The listing builds one solid part. Answer for the finished solid, in the listing's coordinates (mm). A direction names the side the tool comes from. Coordinates: 2 decimals unless noted, no trailing zeros. Order: outer loops, then holes, each group sorted by start corner. A loop starts at its lowest first (then second) coordinate and runs counter-clockwise, first axis right, second up. Notation, with made-up numbers: (48.5, -7) - (74.5, -7) arc R11 ccw to (74.5, 11) - close; hole circle Ø11 at (81, 10.25). An arc over 180 degrees is marked (long way). One line per item, written item: value. Start each with the question number.
```python
from build123d import *

# Parameters (mm, degrees)
F0_R     = 5
F1_DEPTH = 25
F2_DEPTH = 25


with BuildPart() as f1:
    # F0 (on Top) → F1 (new body)
    with BuildSketch(Plane.XY):
        with BuildLine():
            Line((-37.271081, -27.341548), (27.728919, -27.341548))
            Line((27.728919, -27.341548), (27.728919, -12.341548))
            Line((27.728919, -12.341548), (38.254101, 0))
            Line((38.254101, 0), (29.131456, 6.146329))
            Line((29.131456, 6.146329), (16.831115, -3.876174))
            Line((16.831115, -3.876174), (10.514384, 3.876174))
            Line((10.514384, 3.876174), (22.142908, 13.35127))
            Line((22.142908, 13.35127), (14.383989, 22.100874))
            Line((14.383989, 22.100874), (2.728919, 12.658452))
            Line((2.728919, 12.658452), (-7.271081, 12.658452))
            Line((-7.271081, 12.658452), (-7.271081, 2.658452))
            Line((-7.271081, 2.658452), (-12.271081, 2.658452))
            Line((-12.271081, 2.658452), (-12.271081, 12.658452))
            Line((-12.271081, 12.658452), (-32.271081, 12.658452))
            Line((-32.271081, 12.658452), (-32.271081, -7.341548))
            Line((-32.271081, -7.341548), (-37.271081, -7.341548))
            ThreePointArc((-37.271081, -7.341548), (-40.806615, -8.806014), (-42.271081, -12.341548))
            Line((-42.271081, -12.341548), (-42.271081, -22.341548))
            ThreePointArc((-42.271081, -22.341548), (-40.806615, -25.877082), (-37.271081, -27.341548))
        make_face()
        with Locations((-8.769282, -11.614208)):
            Circle(F0_R, mode=Mode.SUBTRACT)
    extrude(amount=F1_DEPTH)

    # F0 (on Top) → F2 (join)
    with BuildSketch(Plane.XY):
        with BuildLine():
            Line((-37.271081, -27.341548), (27.728919, -27.341548))
            Line((27.728919, -27.341548), (27.728919, -12.341548))
            Line((27.728919, -12.341548), (38.254101, 0))
            Line((38.254101, 0), (29.131456, 6.146329))
            Line((29.131456, 6.146329), (16.831115, -3.876174))
            Line((16.831115, -3.876174), (10.514384, 3.876174))
            Line((10.514384, 3.876174), (22.142908, 13.35127))
            Line((22.142908, 13.35127), (14.383989, 22.100874))
            Line((14.383989, 22.100874), (2.728919, 12.658452))
            Line((2.728919, 12.658452), (-7.271081, 12.658452))
            Line((-7.271081, 12.658452), (-7.271081, 2.658452))
            Line((-7.271081, 2.658452), (-12.271081, 2.658452))
            Line((-12.271081, 2.658452), (-12.271081, 12.658452))
            Line((-12.271081, 12.658452), (-32.271081, 12.658452))
            Line((-32.271081, 12.658452), (-32.271081, -7.341548))
            Line((-32.271081, -7.341548), (-37.271081, -7.341548))
            ThreePointArc((-37.271081, -7.341548), (-40.806615, -8.806014), (-42.271081, -12.341548))
            Line((-42.271081, -12.341548), (-42.271081, -22.341548))
            ThreePointArc((-42.271081, -22.341548), (-40.806615, -25.877082), (-37.271081, -27.341548))
        make_face()
        with Locations((-8.769282, -11.614208)):
            Circle(F0_R, mode=Mode.SUBTRACT)
    extrude(amount=F2_DEPTH)


solid = f1.part
```
(1) The part is cut by section A-A on x = -5. Determine the outline of the cut face in (y, z), plus the area to 3 significant figures.
(2) The part is cut by section B-B on y = -1. Determine the outline of the cut face in (x, z), plus the area to 3 significant figures.
(3) For a pull along X with two mould halves and no side action, classify faces 4 (the face through (8.638, 17.446, 12.325)), 5 (the face through (33.8, 3, 12.3)), 6 (the face through (16.25, 8.55, 12.32)), 7 (the face through (-3, -8, 25)) as pulls with the +X half, pulls with the -X half, needs draft (parallel to the pull), parting line crosses it, or undercut.
(4) For faces 1 (the face through (13.717, -0.054, 12.325)), 2 (the face through (-2, 12.658, 12)), 3 (the face through (-10, 2.658, 12)), determine the directions among +Z, -Z, +X, -X, +Y, -Y from which every point of the face is accessible in a straight line to the end or side of a thin tool.
(5) The part is cut by section C-C on z = 9.5. Determine the outline of the cut face in (x, y).
(6) Consider probe 1 along X at (y, z) = (4.5, 5.5) (3 decimals); probe 2 along Y at (x, z) = (-8, 7.75); probe 3 along X at (y, z) = (-13, 20.75). Determine where each line is inside the solid, lowest interval first.
(7) The part is cut by section D-D on y = 5. Determine the outline of the cut face in (x, z).
(8) Flat-ended cylindrical pins translate along their axes: pin 1 Ø6 at (x, z) = (-17.5, 8.5) entering from +Y; pin 2 Ø5 at (x, y) = (5.5, -4.5) entering from -Z; pin 3 Ø12 at (y, z) = (-3.5, 18) entering from -X; pin 4 Ø2 at (y, z) = (-11, 7) entering from -X. Find the tip coordinate at first contact, or state that the pin passes through.
Completed:
1. outline: (-27.34, 0) - (-14.9, 0) - (-14.9, 25) - (-27.34, 25) - close; (-8.33, 0) - (12.66, 0) - (12.66, 25) - (-8.33, 25) - close
1. area: 836 mm2
2. outline: (-32.27, 0) - (14.49, 0) - (14.49, 25) - (-32.27, 25) - close; (20.36, 0) - (37.4, 0) - (37.4, 25) - (20.36, 25) - close
2. area: 1,590 mm2
3. face 4: pulls with the -X half
3. face 5: pulls with the +X half
3. face 6: undercut
3. face 7: needs draft
4. face 1: +Z, -Z
4. face 2: +Z, -Z, -X, +Y
4. face 3: +Z, -Z, +Y
5. outline: (-42.27, -22.34) arc R5 ccw to (-37.27, -27.34) - (27.73, -27.34) - (27.73, -12.34) - (38.25, 0) - (29.13, 6.15) - (16.83, -3.88) - (10.51, 3.88) - (22.14, 13.35) - (14.38, 22.1) - (2.73, 12.66) - (-7.27, 12.66) - (-7.27, 2.66) - (-12.27, 2.66) - (-12.27, 12.66) - (-32.27, 12.66) - (-32.27, -7.34) - (-37.27, -7.34) arc R5 ccw to (-42.27, -12.34) - close; hole circle Ø10 at (-8.77, -11.61)
6. probe 1: x = -32.271 to -12.271, -7.271 to 11.28, 27.111 to 31.575
6. probe 2: y = -27.34 to -16.55, -6.67 to 2.66
6. probe 3: x = -42.27 to -13.57, -3.97 to 27.73
7. outline: (-32.27, 0) - (-12.27, 0) - (-12.27, 25) - (-32.27, 25) - close; (-7.27, 0) - (11.89, 0) - (11.89, 25) - (-7.27, 25) - close; (27.72, 0) - (30.83, 0) - (30.83, 25) - (27.72, 25) - close
8. pin 1: stops at y = 12.66
8. pin 2: stops at z = 0
8. pin 3: stops at x = -41.39
8. pin 4: stops at x = -42.26
